Verification items for the finished model (mm, model axes). Face numbers are marked on the shaded views. A direction names the side the tool comes from. Round coordinates to 2 decimals unless told otherwise and drop trailing zeros. Loops run counter-clockwise (first coordinate to the right, second up) from the corner with the lowest first, then second, coordinate; pieces in that order, holes last. Notation, with made-up numbers: (35.25, -16) -> (58.25, -16) arc R15 cw to (58.25, -5) -> close; hole circle Ø8 at (-32.75, 24). An arc over 180 degrees is marked (long way). Write item = value, one per line. Start each with the question number.
```python
from build123d import *

# Parameters (mm, degrees)
CUT_EXTRUDE2_START = -7
SKETCH4_R          = 5
SKETCH4_R_2        = 3.8
CUT_EXTRUDE2_DEPTH = 7
SKETCH6_R          = 5
SKETCH6_R_2        = 3.8
CUT_EXTRUDE6_DEPTH = 12
CUT_EXTRUDE5_DEPTH = 5


with BuildPart() as part:
    # Sketch2 → Revolve1 (revolve)
    with BuildSketch(Plane(origin=(0, 0, 0), x_dir=(1, 0, 0), z_dir=(0, 1, 0))):
        Polygon((30, -5), (-30, -5), (-30, 0), (-19.977940469, 0), (-19.25, -2), (-16.75, -2), (-16.022059531, 0), (-7.977940469, 0), (-7.25, -2), (-4.75, -2), (-4.022059531, 0), (4.022059531, 0), (4.75, -2), (7.25, -2), (7.977940469, 0), (16.022059531, 0), (16.75, -2), (19.25, -2), (19.977940469, 0), (30, 0), align=None)
    revolve(axis=Axis((30, 0, 5), (-1, 0, 0)))

    # Sketch4 → Cut-Extrude2 (cut)
    with BuildSketch(Plane.ZY.offset(30).offset(CUT_EXTRUDE2_START)):
        with Locations(Location((5, 0, 0), (0, 0, 180))):
            Circle(SKETCH4_R)
        with Locations((5, 0)):
            Circle(SKETCH4_R_2, mode=Mode.SUBTRACT)
    extrude(amount=CUT_EXTRUDE2_DEPTH, mode=Mode.SUBTRACT)

    # Sketch6 → Cut-Extrude6 (cut)
    with BuildSketch(Plane(origin=(30, 0, 0), x_dir=(0, 0, -1), z_dir=(1, 0, 0))):
        with Locations((-5, 0)):
            Circle(SKETCH6_R)
        with Locations(Location((-5, 0, 0), (0, 0, 180))):
            Circle(SKETCH6_R_2, mode=Mode.SUBTRACT)
    extrude(amount=-CUT_EXTRUDE6_DEPTH, mode=Mode.SUBTRACT)

    # Sketch5 → Cut-Extrude5 (cut)
    with BuildSketch(Plane(origin=(30, 0, 0), x_dir=(0, 0, -1), z_dir=(1, 0, 0))):
        with BuildLine():
            Line((-8.307550461, 1.870858078), (-1.692449539, 1.870858078))
            ThreePointArc((-1.692449539, 1.870858078), (-5, 3.8), (-8.307550461, 1.870858078))
        make_face()
    extrude(amount=-CUT_EXTRUDE5_DEPTH, mode=Mode.SUBTRACT)


solid = part.part
```
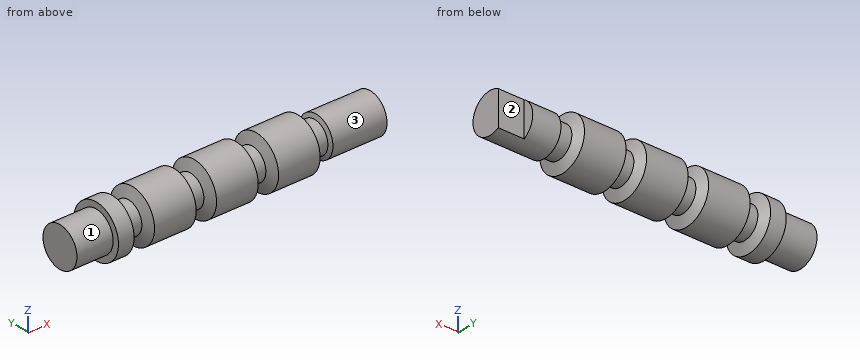
(1) Section check B-B on x = 11. Enter the section's corners in (y, z).
(2) Access from +Z, -Z, +X, -X, +Y, -Y to the whole of each face (thin tool, end or side, straight path). Record for the marked faces 1, 2 and 3.
(3) Scan lines: line 1 (X direction, y = 4.25, z = 5.5); line 2 (X direction, y = -3.5, z = 5.5); line 3 (X direction, y = 3.5, z = 4.25). Record each from-to range of solid material in increasing order. Write a range as [from, to].
(4) Depth check by flat-ended pin: pin 1 Ø3 at (y, z) = (-3.5, 7) entering from -X; pin 2 Ø3 at (x, y) = (-17, -3.5) entering from +Z; pin 3 Ø6 at (x, z) = (-20, 1) entering from +Y; pin 4 Ø1.5 at (x, z) = (28.5, 4.5) entering from +Y. Enter the tip coordinate at first touch or a pass-through.
(5) Section check A-A on x = -25.5. Enter the section's corners in (y, z), then the cut area to 3 significant figures.
Computed values:
q1.outline = circle Ø10 at (0, 5)
q2.face_1 = -X
q2.face_2 = +Z, -Z, +X, +Y
q2.face_3 = +X
q3.line_1 = [-23, -19.72], [-16.28, -7.72], [-4.28, 4.28], [7.72, 16.28]
q3.line_2 = [-30, -19.44], [-16.56, -7.44], [-4.56, 4.56], [7.44, 16.56], [19.44, 30]
q3.line_3 = [-30, -19.46], [-16.54, -7.46], [-4.54, 4.54], [7.46, 16.54], [19.46, 25]
q4.pin_1 = -30
q4.pin_2 = 9.41
q4.pin_3 = 4.9
q4.pin_4 = 1.87
q5.outline = circle Ø7.6 at (0, 5)
q5.area = 45.4 mm²
